```python
from build123d import *

# Parameters (mm, degrees)
BOSS_EXTRUDE1_DEPTH = 1.6
SKETCH1_5_R         = 5.5
CUT_EXTRUDE3_DEPTH  = 59.711668346


with BuildPart() as part:
    # Sketch1 → Boss-Extrude1 (new body)
    with BuildSketch(Plane.XY):
        with BuildLine():
            Line((-3.429, -22.169410702), (-3.429, -26.178))
            ThreePointArc((-3.429, -26.178), (-3.136106781, -26.885106781), (-2.429, -27.178))
            Line((-2.429, -27.178), (2.429, -27.178))
            ThreePointArc((2.429, -27.178), (3.136106781, -26.885106781), (3.429, -26.178))
            Line((3.429, -26.178), (3.429, -22.22966812))
            ThreePointArc((3.429, -22.22966812), (4.826254657, -19.693685595), (7.716471578, -19.519978666))
            ThreePointArc((7.716471578, -19.519978666), (9.379032197, -20.419956769), (10.937907763, -21.489524611))
            ThreePointArc((10.937907763, -21.489524611), (16.695290309, -26.175210804), (22.169453406, -31.188856909))
            ThreePointArc((22.169453406, -31.188856909), (23.117301861, -32.459556006), (23.619723106, -33.963107063))
            ThreePointArc((23.619723106, -33.963107063), (38.862466656, -38.865455055), (33.967276916, -23.620411133))
            ThreePointArc((33.967276916, -23.620411133), (32.455427267, -23.112806715), (31.180313141, -22.154978144))
            ThreePointArc((31.180313141, -22.154978144), (27.47385025, -18.084321842), (23.999156064, -13.81412159))
            ThreePointArc((23.999156064, -13.81412159), (20.509860624, -7.295108734), (19.304, 0))
            ThreePointArc((19.304, 0), (20.509860624, 7.295108734), (23.999156064, 13.81412159))
            ThreePointArc((23.999156064, 13.81412159), (27.47385025, 18.084321842), (31.180313141, 22.154978144))
            ThreePointArc((31.180313141, 22.154978144), (32.455427267, 23.112806715), (33.967276916, 23.620411133))
            ThreePointArc((33.967276916, 23.620411133), (38.861014354, 38.866906343), (23.61905648, 33.959055239))
            ThreePointArc((23.61905648, 33.959055239), (23.121622823, 32.463531472), (22.183380489, 31.19714571))
            ThreePointArc((22.183380489, 31.19714571), (17.368920037, 26.656724902), (12.387395689, 22.300250899))
            ThreePointArc((12.387395689, 22.300250899), (11.895164251, 21.899521015), (11.389978134, 21.515251299))
            ThreePointArc((11.389978134, 21.515251299), (6.171223513, 21.083006766), (3.429, 25.544222445))
            Line((3.429, 25.544222445), (3.429, 25.6764))
            ThreePointArc((3.429, 25.6764), (2.43210864, 28.08310864), (0.0254, 29.08))
            Line((0.0254, 29.08), (-0.0254, 29.08))
            ThreePointArc((-0.0254, 29.08), (-2.43210864, 28.08310864), (-3.429, 25.6764))
            Line((-3.429, 25.6764), (-3.429, 25.544222445))
            ThreePointArc((-3.429, 25.544222445), (-6.171223513, 21.083006766), (-11.389978134, 21.515251299))
            ThreePointArc((-11.389978134, 21.515251299), (-11.895164251, 21.899521015), (-12.387395689, 22.300250899))
            ThreePointArc((-12.387395689, 22.300250899), (-17.368920037, 26.656724902), (-22.183380489, 31.19714571))
            ThreePointArc((-22.183380489, 31.19714571), (-23.121622823, 32.463531472), (-23.61905648, 33.959055239))
            ThreePointArc((-23.61905648, 33.959055239), (-38.861014354, 38.866906343), (-33.967276916, 23.620411133))
            ThreePointArc((-33.967276916, 23.620411133), (-32.455427267, 23.112806715), (-31.180313141, 22.154978144))
            ThreePointArc((-31.180313141, 22.154978144), (-27.47385025, 18.084321842), (-23.999156064, 13.81412159))
            ThreePointArc((-23.999156064, 13.81412159), (-20.509860624, 7.295108734), (-19.304, 0))
            ThreePointArc((-19.304, 0), (-20.509860624, -7.295108734), (-23.999156064, -13.81412159))
            ThreePointArc((-23.999156064, -13.81412159), (-27.47385025, -18.084321842), (-31.180313141, -22.154978144))
            ThreePointArc((-31.180313141, -22.154978144), (-32.455427267, -23.112806715), (-33.967276916, -23.620411133))
            ThreePointArc((-33.967276916, -23.620411133), (-38.862466656, -38.865455055), (-23.619723106, -33.963107063))
            ThreePointArc((-23.619723106, -33.963107063), (-23.117301861, -32.459556006), (-22.169453406, -31.188856909))
            ThreePointArc((-22.169453406, -31.188856909), (-16.695290309, -26.175210804), (-10.937907763, -21.489524611))
            ThreePointArc((-10.937907763, -21.489524611), (-9.414925724, -20.426362093), (-7.803463878, -19.502793172))
            ThreePointArc((-7.803463878, -19.502793172), (-4.867492977, -19.607829975), (-3.429, -22.169410702))
        make_face()
    extrude(amount=BOSS_EXTRUDE1_DEPTH)

    # Sketch1<5> → Cut-Extrude3 (cut, through all)
    with BuildSketch(Plane.XY):
        with Locations((-32.5, -32.5)):
            Circle(SKETCH1_5_R)
        with Locations((32.5, -32.5)):
            Circle(SKETCH1_5_R)
        with Locations((32.5, 32.5)):
            Circle(SKETCH1_5_R)
        with Locations((-32.5, 32.5)):
            Circle(SKETCH1_5_R)
        with BuildLine():
            ThreePointArc((-24.998680714, -27.527052285), (-24.266539251, -27.975169466), (-23.452541635, -27.702684585))
            ThreePointArc((-23.452541635, -27.702684585), (-17.751335536, -22.602028101), (-11.761197607, -17.84401432))
            ThreePointArc((-11.761197607, -17.84401432), (-11.363038546, -17.168840008), (-11.563944828, -16.411193879))
            ThreePointArc((-11.563944828, -16.411193879), (-13.962913518, -13.697220596), (-16.710750131, -11.337115576))
            ThreePointArc((-16.710750131, -11.337115576), (-17.483496193, -11.148963344), (-18.155018506, -11.575103607))
            ThreePointArc((-18.155018506, -11.575103607), (-22.713350188, -17.692311571), (-27.713994469, -23.453576864))
            ThreePointArc((-27.713994469, -23.453576864), (-27.981074308, -24.266291585), (-27.532770213, -24.994893189))
            ThreePointArc((-27.532770213, -24.994893189), (-26.138464304, -26.133614559), (-24.998680714, -27.527052285))
        make_face()
        with BuildLine():
            ThreePointArc((18.155018506, -11.575103607), (17.483496193, -11.148963344), (16.710750131, -11.337115576))
            ThreePointArc((16.710750131, -11.337115576), (13.962913518, -13.697220596), (11.563944828, -16.411193879))
            ThreePointArc((11.563944828, -16.411193879), (11.363038546, -17.168840008), (11.761197607, -17.84401432))
            ThreePointArc((11.761197607, -17.84401432), (17.751335536, -22.602028101), (23.452541635, -27.702684585))
            ThreePointArc((23.452541635, -27.702684585), (24.266539251, -27.975169466), (24.998680714, -27.527052285))
            ThreePointArc((24.998680714, -27.527052285), (26.138464304, -26.133614559), (27.532770213, -24.994893189))
            ThreePointArc((27.532770213, -24.994893189), (27.981074308, -24.266291585), (27.713994469, -23.453576864))
            ThreePointArc((27.713994469, -23.453576864), (22.713350188, -17.692311571), (18.155018506, -11.575103607))
        make_face()
        with BuildLine():
            ThreePointArc((-12.074975691, 17.380952209), (-17.927124595, 22.331716527), (-23.562984675, 27.527368101))
            ThreePointArc((-23.562984675, 27.527368101), (-24.368188535, 27.806201558), (-25.102498374, 27.37389332))
            ThreePointArc((-25.102498374, 27.37389332), (-26.204243006, 26.068558181), (-27.532770213, 24.994893189))
            ThreePointArc((-27.532770213, 24.994893189), (-27.981074308, 24.266291585), (-27.713994469, 23.453576864))
            ThreePointArc((-27.713994469, 23.453576864), (-22.713350188, 17.692311571), (-18.155018506, 11.575103607))
            ThreePointArc((-18.155018506, 11.575103607), (-17.483496193, 11.148963344), (-16.710750131, 11.337115576))
            ThreePointArc((-16.710750131, 11.337115576), (-14.170722957, 13.494587833), (-11.922695283, 15.954830943))
            ThreePointArc((-11.922695283, 15.954830943), (-11.704234617, 16.699348887), (-12.074975691, 17.380952209))
        make_face()
        with BuildLine():
            ThreePointArc((25.102498374, 27.37389332), (24.368188535, 27.806201558), (23.562984675, 27.527368101))
            ThreePointArc((23.562984675, 27.527368101), (17.927124595, 22.331716527), (12.074975691, 17.380952209))
            ThreePointArc((12.074975691, 17.380952209), (11.704234617, 16.699348887), (11.922695283, 15.954830943))
            ThreePointArc((11.922695283, 15.954830943), (14.170722957, 13.494587833), (16.710750131, 11.337115576))
            ThreePointArc((16.710750131, 11.337115576), (17.483496193, 11.148963344), (18.155018506, 11.575103607))
            ThreePointArc((18.155018506, 11.575103607), (22.713350188, 17.692311571), (27.713994469, 23.453576864))
            ThreePointArc((27.713994469, 23.453576864), (27.981074308, 24.266291585), (27.532770213, 24.994893189))
            ThreePointArc((27.532770213, 24.994893189), (26.204243006, 26.068558181), (25.102498374, 27.37389332))
        make_face()
    extrude(amount=CUT_EXTRUDE3_DEPTH, mode=Mode.SUBTRACT)


solid = part.part
```
Geometry: final body of the model. Coordinates: model frame, mm. A direction names the side the tool comes from. Coordinates: 2 decimals unless noted, no trailing zeros. Loops run counter-clockwise (first coordinate to the right, second up) from the corner with the lowest first, then second, coordinate; pieces in that order, holes last. Notation, with made-up numbers: (-32.5, -4) -> (13.5, -4) arc R8 cw to (13.5, 7) -> close; hole circle Ø4 at (-18, -34). An arc over 180 degrees is marked (long way). Use a Markdown table: item, result. Add a question column.
(1) Mould query, pull axis X, two halves, no side actions, for faces 1 (the cylindrical face through (27.52, -18.14, 0.79)), 2 (the cylindrical face through (-39.05, -38.67, 0.79)), 3 (the flat face through (-1, 1, 0)), 4 (the cylindrical face through (-27.4, -18, 0.8)). Classes: pulls with the +X half, pulls with the -X half, needs draft (parallel to the pull), parting line crosses it, or undercut.
(2) Section query A-A, the plane y = 32.5. Return loops of the section in (x, z).
(3) Pin query (flat end, axial travel): pin 1 Ø3 at (x, y) = (-7, -11) entering from -Z; pin 2 Ø10 at (x, y) = (-32.5, -32.5) entering from +Z; pin 3 Ø0.5 at (x, z) = (-1, 1) entering from -Y. Return the tip coordinate at first contact, or that it passes through.
(4) Section query C-C, the plane z = 0.6. State how many separate pieces and enclosed holes the cut face has, plus the area to 3 significant figures.
(5) Access query for faces 5 (the cylindrical face through (-13.93, -13.73, 0.79)), 6 (the cylindrical face through (2.458, 28.057, 0.789)), 7 (the cylindrical face through (16.62, -26.11, 0.79)). Directions: +Z, -Z, +X, -X, +Y, -Y. A direction counts if a zero-diameter tool reaches every point of the face in a straight line with its end or side. Return the directions, or none.
(6) Section query D-D, the plane y = -6. Return loops of the section in (x, z), plus the area to 3 significant figures.
(7) Line query: line 1 along X through (y, z) = (-32.5, 1); line 2 along X through (y, z) = (-36.5, 1.05). Output: solid intervals per line, ascending.
Answer:
| question | item | result |
|---|---|---|
| 1 | face 1 | pulls with the +X half |
| 1 | face 2 | undercut |
| 1 | face 3 | needs draft |
| 1 | face 4 | pulls with the -X half |
| 2 | outline | (-41.5, 0) -> (-38, 0) -> (-38, 1.6) -> (-41.5, 1.6) -> close; (-27, 0) -> (-23.14, 0) -> (-23.14, 1.6) -> (-27, 1.6) -> close; (23.14, 0) -> (27, 0) -> (27, 1.6) -> (23.14, 1.6) -> close; (38, 0) -> (41.5, 0) -> (41.5, 1.6) -> (38, 1.6) -> close |
| 3 | pin 1 | stops at z = 0 |
| 3 | pin 2 | passes through |
| 3 | pin 3 | stops at y = -27.18 |
| 4 | separate pieces | 1 |
| 4 | enclosed holes | 8 |
| 4 | area | 2,590 mm^2 |
| 5 | face 5 | +Z, -Z |
| 5 | face 6 | +Z, -Z, +Y |
| 5 | face 7 | +Z, -Z, -Y |
| 6 | outline | (-20.11, 0) -> (20.11, 0) -> (20.11, 1.6) -> (-20.11, 1.6) -> close |
| 6 | area | 64.4 mm^2 |
| 7 | line 1 | x = -41.5 to -38, -27 to -23.14, 23.14 to 27, 38 to 41.5 |
| 7 | line 2 | x = -40.56 to -36.27, -28.73 to -24.44, 24.44 to 28.73, 36.27 to 40.56 |
